Input: part model. Units: mm. Frame: model coordinates. A direction names the side the tool comes from. Coordinates: 2 decimals unless noted, no trailing zeros. Loops run counter-clockwise (first coordinate to the right, second up) from the corner with the lowest first, then second, coordinate; pieces in that order, holes last. Notation, with made-up numbers: M -9.75,86.5 L 12.25,86.5 A24 cw 12.25,98.5 Z; hole C 71.5,72.25 d7. An arc over 180 degrees is marked long. Use a Markdown table: item, result. Add a question column.
1. Section B-B on y = -9. Output: boundary loops of the cut face in (x, z).
2. Set-up query: faces 1 (the cylindrical face through (0, 3, 49)), 2 (the flat face through (0, 12.5, 17)). Return all of +Z, -Z, +X, -X, +Y, -Y with unobstructed straight access to the full face (end or side cutting, diameter ignored); none if empty.
3. Section A-A on x = 0. Output: boundary loops of the cut face in (y, z), then the cut area to 3 significant figures.
4. Pin query (flat end, axial travel): pin 1 (12 mm diameter, centred on y = 1.5, z = 51.5, fed in from -X); pin 2 (5 mm diameter, centred on y = -9.5, z = 39, fed in from +X); pin 3 (3 mm diameter, centred on x = -2, z = 28.5, fed in from +Y). Return the tip coordinate at first contact, or that it passes through.
5. Line query: L1, parallel to Z at x = 2.6, y = 7; L2, parallel to Z at x = -2.6, y = -3.5; L3, parallel to Y at x = -2.1, z = 26.5 (3 decimals). Output: solid intervals per line, ascending. Write a range as [from, to].
6. Section D-D on x = 2.3. Output: boundary loops of the cut face in (y, z), then the cut area to 3 significant figures.
7. Section C-C on z = 46. Output: boundary loops of the cut face in (x, y).
```python
from build123d import *

# Parameters (mm, degrees)
F1_DEPTH = 25
F2_DEPTH = 65
F4_DEPTH = 3
F5_DEPTH = 10


with BuildPart() as f1:
    # F0 (on Top) → F1 (new body)
    with BuildSketch(Plane.XY):
        with BuildLine():
            ThreePointArc((-3, 0), (0, 3), (3, 0))
            Line((3, 0), (3, 12.5))
            Line((3, 12.5), (-3, 12.5))
            Line((-3, 12.5), (-3, 0))
        make_face()
    extrude(amount=F1_DEPTH)



with BuildPart() as f1b:
    # F0 (on Top) → F1, piece 2 (new body)
    with BuildSketch(Plane.XY):
        with BuildLine():
            Line((3, -12.5), (3, 0))
            ThreePointArc((3, 0), (0, -3), (-3, 0))
            Line((-3, 0), (-3, -12.5))
            Line((-3, -12.5), (3, -12.5))
        make_face()
    extrude(amount=F1_DEPTH)


with BuildPart() as f1_1:
    add(f1.part)

    add(f1b.part)  # F2 merges F1b
    # F0 (on Top) → F2 (join)
    with BuildSketch(Plane.XY):
        with BuildLine():
            ThreePointArc((-3, 0), (0, -3), (3, 0))
            ThreePointArc((3, 0), (0, 3), (-3, 0))
        make_face()
    extrude(amount=F2_DEPTH)

    # F3 (on Right) → F4 (join, symmetric)
    with BuildSketch(Plane.YZ):
        Polygon((-12.5, 25), (0, 25), (0, 55), align=None)
    extrude(amount=F4_DEPTH, both=True)

    # F0 (on Top) → F5 (cut)
    with BuildSketch(Plane.XY):
        with BuildLine():
            ThreePointArc((-3, 0), (0, 3), (3, 0))
            Line((3, 0), (3, 12.5))
            Line((3, 12.5), (-3, 12.5))
            Line((-3, 12.5), (-3, 0))
        make_face()
        with BuildLine():
            ThreePointArc((-3, 0), (0, -3), (3, 0))
            ThreePointArc((3, 0), (0, 3), (-3, 0))
        make_face()
        with BuildLine():
            Line((3, -12.5), (3, 0))
            ThreePointArc((3, 0), (0, -3), (-3, 0))
            Line((-3, 0), (-3, -12.5))
            Line((-3, -12.5), (3, -12.5))
        make_face()
    extrude(amount=F5_DEPTH, mode=Mode.SUBTRACT)


solid = f1_1.part
```
Answers below:
| question | item | result |
|---|---|---|
| 1 | outline | M -3,10 L 3,10 L 3,33.4 L -3,33.4 Z |
| 2 | face 1 | +Z |
| 2 | face 2 | +Z, -Z, +X, -X, +Y |
| 3 | outline | M -12.5,10 L 12.5,10 L 12.5,25 L 3,25 L 3,65 L -3,65 L -3,47.8 L -12.5,25 Z |
| 3 | area | 723 mm² |
| 4 | pin 1 | stops at x = -3 |
| 4 | pin 2 | passes through |
| 4 | pin 3 | stops at y = 2.96 |
| 5 | L1 | z = [10, 25] |
| 5 | L2 | z = [10, 46.6] |
| 5 | L3 | y = [-11.875, 2.142] |
| 6 | outline | M -12.5,10 L 12.5,10 L 12.5,25 L 1.93,25 L 1.93,65 L -1.93,65 L -1.93,50.38 L -12.5,25 Z |
| 6 | area | 663 mm² |
| 7 | outline | M -3,-3.75 L 3,-3.75 L 3,0 A3 ccw -3,0 Z |
